For this review, take the finished solid that the model builds, in its own axes (mm). Give positions to 0.01 mm unless a question says otherwise; leave off trailing zeros. Order: outer loops, then holes, each group sorted by start corner. A loop starts at its lowest first (then second) coordinate and runs counter-clockwise, first axis right, second up. Notation, with made-up numbers: (-7.75, -27.75) - (51.25, -27.75) arc R18 cw to (51.25, -14.75) - close; hole circle Ø7 at (44, 35.25). An arc over 180 degrees is marked (long way). Use a Markdown table: item, result. Add a question column.
1) We need section C-C on z = 73.5. Write out the cut boundary in (x, y), then the cut area to 3 significant figures.
2) We need section B-B on y = 250. Write out the cut boundary in (x, z).
3) Clearance check with flat-ended pins moving along their axes: P1, Ø1, axis at y = 312, z = 71, coming from the -X side; P2, Ø8, axis at x = 61.5, z = 205, coming from the +Y side; P3, Ø10, axis at y = 127.5, z = 195, coming from the +X side. State where each tip first meets the part, or that it passes through.
4) We need section A-A on x = 85. Write out the cut boundary in (y, z) (1 decimal), then the cut area to 3 significant figures.
5) We need section D-D on y = 180. Write out the cut boundary in (x, z), then the cut area to 3 significant figures.
6) Wall thickness on L1, parallel to Z at x = 15, y = 88.5; L2, parallel to Y at x = -193, z = 142.5; L3, parallel to X at y = 309, z = 65: over which ranges is each line inside the solid? List them lowest first.
```python
from build123d import *

# Parameters (mm, degrees)
F2_DEPTH = 431.8
F3_DEPTH = 300
F5_DEPTH = 335.336541


with BuildPart() as f2:
    # F0 (on Front) → F2 (new body)
    with BuildSketch(Plane.XZ):
        with BuildLine():
            ThreePointArc((-215.083709, 28.186797), (-206.182504, 20.924757), (-194.992326, 18.326948))
            Line((-194.992326, 18.326948), (194.992326, 18.326948))
            ThreePointArc((194.992326, 18.326948), (206.182504, 20.924757), (215.083709, 28.186797))
            Line((215.083709, 28.186797), (291.649465, 127.176309))
            ThreePointArc((291.649465, 127.176309), (295.594316, 134.505526), (296.958081, 142.71646))
            Line((296.958081, 142.71646), (296.958081, 277.847902))
            ThreePointArc((296.958081, 277.847902), (294.447383, 288.858799), (287.411636, 297.692921))
            Line((287.411636, 297.692921), (243.500706, 332.771967))
            ThreePointArc((243.500706, 332.771967), (236.046451, 336.898009), (227.647151, 338.326948))
            Line((227.647151, 338.326948), (-227.647151, 338.326948))
            ThreePointArc((-227.647151, 338.326948), (-236.046451, 336.898009), (-243.500706, 332.771967))
            Line((-243.500706, 332.771967), (-283.495474, 300.821419))
            ThreePointArc((-283.495474, 300.821419), (-290.531221, 291.987297), (-293.041919, 280.9764))
            Line((-293.041919, 280.9764), (-293.041919, 128.976569))
            Line((-293.041919, 128.976569), (-215.083709, 28.186797))
        make_face()
    extrude(amount=-F2_DEPTH)

    # F1 (on Right) → F3 (intersect, symmetric)
    with BuildSketch(Plane.YZ):
        with BuildLine():
            Line((80.317164, 15.33554), (122.591108, 15.33554))
            Line((122.591108, 15.33554), (341.597618, 15.33554))
            ThreePointArc((341.597618, 15.33554), (372.701891, 25.971325), (390.78182, 53.425138))
            Line((390.78182, 53.425138), (416.052516, 151.212684))
            ThreePointArc((416.052516, 151.212684), (417.546314, 167.441665), (413.824101, 183.308498))
            Line((413.824101, 183.308498), (380.432576, 264.190209))
            ThreePointArc((380.432576, 264.190209), (376.455207, 270.772931), (370.689926, 275.863436))
            Line((370.689926, 275.863436), (308.221791, 316.021523))
            ThreePointArc((308.221791, 316.021523), (303.123356, 318.542104), (297.591884, 319.86505))
            Line((297.591884, 319.86505), (173.547573, 335.145001))
            ThreePointArc((173.547573, 335.145001), (171.997825, 335.287861), (170.442237, 335.33554))
            Line((170.442237, 335.33554), (122.591108, 335.33554))
            Line((122.591108, 335.33554), (90.687651, 335.33554))
            ThreePointArc((90.687651, 335.33554), (77.918617, 331.892584), (68.611255, 322.497098))
            Line((68.611255, 322.497098), (0, 201.915771))
            Line((0, 201.915771), (0, 118.959656))
            ThreePointArc((0, 118.959656), (0.696999, 113.050193), (2.749745, 107.465051))
            Line((2.749745, 107.465051), (34.218363, 45.45577))
            ThreePointArc((34.218363, 45.45577), (37.734355, 40.245886), (42.421994, 36.058868))
            Line((42.421994, 36.058868), (65.87054, 19.844034))
            ThreePointArc((65.87054, 19.844034), (72.750271, 16.488847), (80.317164, 15.33554))
        make_face()
    extrude(amount=F3_DEPTH, both=True, mode=Mode.INTERSECT)

    # F4 (on Top) → F5 (intersect, through all)
    with BuildSketch(Plane.XY):
        Polygon((-166.86368, 0), (0, 0), (166.86368, 0), (262.060732, 66.595584), (297.64843, 145.778194), (297.64843, 268.555701), (190.885365, 418.913692), (0, 418.913692), (-190.885365, 418.913692), (-297.64843, 268.555701), (-297.64843, 145.778194), (-262.060732, 66.595584), align=None)
    extrude(amount=F5_DEPTH, mode=Mode.INTERSECT)


solid = f2.part
```
Checked values:
| question | item | result |
|---|---|---|
| 1 | outline | (-250.13, 58.25) - (-195.43, 19.99) - (195.43, 19.99) - (250.13, 58.25) - (250.13, 335.47) - (207.18, 395.97) - (-207.18, 395.97) - (-250.13, 335.47) - close |
| 1 | area | 183,000 mm² |
| 2 | outline | (-293.04, 128.98) - (-215.08, 28.19) arc R25.4 ccw to (-194.99, 18.33) - (194.99, 18.33) arc R25.4 ccw to (215.08, 28.19) - (291.65, 127.18) arc R25.4 ccw to (296.96, 142.72) - (296.96, 277.85) arc R25.4 ccw to (287.41, 297.69) - (252.32, 325.73) - (-252.32, 325.73) - (-283.5, 300.82) arc R25.4 ccw to (-293.04, 280.98) - close |
| 3 | P1 | x = -248.59 |
| 3 | P2 | y = 406.52 |
| 3 | P3 | x = 291.68 |
| 4 | outline | (0, 119) arc R25.4 ccw to (2.7, 107.5) - (34.2, 45.5) arc R25.4 ccw to (42.4, 36.1) - (65.9, 19.8) arc R25.4 ccw to (68.4, 18.3) - (358.8, 18.3) arc R50.8 ccw to (390.8, 53.4) - (416.1, 151.2) arc R50.8 ccw to (413.8, 183.3) - (380.4, 264.2) arc R25.4 ccw to (370.7, 275.9) - (308.2, 316) arc R25.4 ccw to (297.6, 319.9) - (173.5, 335.1) arc R25.4 ccw to (170.4, 335.3) - (90.7, 335.3) arc R25.4 ccw to (68.6, 322.5) - (0, 201.9) - close |
| 4 | area | 114,000 mm² |
| 5 | outline | (-293.04, 128.98) - (-215.08, 28.19) arc R25.4 ccw to (-194.99, 18.33) - (194.99, 18.33) arc R25.4 ccw to (215.08, 28.19) - (291.65, 127.18) arc R25.4 ccw to (296.96, 142.72) - (296.96, 277.85) arc R25.4 ccw to (287.41, 297.69) - (243.5, 332.77) arc R25.4 ccw to (241.29, 334.35) - (-241.29, 334.35) arc R25.4 ccw to (-243.5, 332.77) - (-283.5, 300.82) arc R25.4 ccw to (-293.04, 280.98) - close |
| 5 | area | 174,000 mm² |
| 6 | L1 | 18.33 to 335.24 |
| 6 | L2 | 18.28 to 413.8 |
| 6 | L3 | -243.56 to 243.56 |
